from build123d import *

# Parameters (mm, degrees)
Y_KSEKLIK_EKSTR_ZYON1_DEPTH = 15
KES_EKSTR_ZYON1_DEPTH       = 10
IZIM4_W                     = 15
IZIM4_H                     = 10
KES_EKSTR_ZYON2_DEPTH       = 10


with BuildPart() as part:
    # Çizim2 → Yükseklik-Ekstrüzyon1 (new, symmetric)
    with BuildSketch(Plane.XY):
        Polygon((0, 0), (0, 30), (-10, 30), (-10, 10), (-40, 10), (-40, 0), align=None)
    extrude(amount=Y_KSEKLIK_EKSTR_ZYON1_DEPTH, both=True)

    # Çizim3 → Kes-Ekstrüzyon1 (cut)
    with BuildSketch(Plane(origin=(0, 0, 0), x_dir=(1, 0, 0), z_dir=(0, 1, 0))):
        Polygon((-40, 15), (-25, 15), (-40, 7.5), align=None)
        Polygon((-25, -15), (-40, -7.5), (-40, -15), align=None)
    extrude(amount=KES_EKSTR_ZYON1_DEPTH, mode=Mode.SUBTRACT)

    # Çizim4 → Kes-Ekstrüzyon2 (cut)
    with BuildSketch(Plane.ZY.offset(10)):
        with Locations((7.5, 25)):
            Rectangle(IZIM4_W, IZIM4_H)
    extrude(amount=-KES_EKSTR_ZYON2_DEPTH, mode=Mode.SUBTRACT)


solid = part.part
The model under review builds one solid part; all positions refer to its coordinate system, in mm. A direction names the side the tool comes from. Give positions to 0.01 mm unless a question says otherwise; leave off trailing zeros. Loops run counter-clockwise (first coordinate to the right, second up) from the corner with the lowest first, then second, coordinate; pieces in that order, holes last. Notation, with made-up numbers: (-7, 67) -> (38, 67) arc R10 ccw to (38, 75) -> close; hole circle Ø1 at (-40, 36.5). An arc over 180 degrees is marked (long way). Put each result on its own line as item: value. Start each with the question number.
1. We need section D-D on y = 12. State the section outline as (x, z) points.
2. We need section B-B on y = 4.5. State the section outline as (x, z) points.
3. We need section A-A on z = 11.75. State the section outline as (x, y) points, then the cut area to 3 significant figures.
4. We need section C-C on x = -25.5. State the section outline as (y, z) points.
5. Wall thickness on probe 1 along Y at (x, z) = (-38, -3); probe 2 along X at (y, z) = (27.5, -10.25); probe 3 along Y at (x, z) = (-1.5, 12.75): over which ranges is each line inside the solid? List them lowest first.
6. For faces 1 (the face through (-5, 25, 0)), 2 (the face through (-25, 10, 0)), 3 (the face through (-10, 8, 15)), list the 3-axis set-ups (+Z, -Z, +X, -X, +Y, -Y) from which the entire face can be reached by the end or side of a thin tool; tool diameter is ignored.
7. Clearance check with flat-ended pins moving along their axes: P1, Ø6, axis at y = 16, z = -4, coming from the +X side; P2, Ø3, axis at x = -5, y = 24, coming from the +Z side; P3, Ø10, axis at y = 19, z = 3.5, coming from the -X side; P4, Ø9, axis at x = -18, z = 4.5, coming from the +Y side. State where each tip first meets the part, or that it passes through.
Determined:
1. outline: (-10, -15) -> (0, -15) -> (0, 15) -> (-10, 15) -> close
2. outline: (-40, -7.5) -> (-25, -15) -> (0, -15) -> (0, 15) -> (-25, 15) -> (-40, 7.5) -> close
3. outline: (-31.5, 0) -> (0, 0) -> (0, 20) -> (-10, 20) -> (-10, 10) -> (-31.5, 10) -> close
3. area: 415 mm^2
4. outline: (0, -14.75) -> (10, -14.75) -> (10, 14.75) -> (0, 14.75) -> close
5. probe 1: 0 to 10
5. probe 2: -10 to 0
5. probe 3: 0 to 20
6. face 1: +Z, +X, -X, +Y
6. face 2: +Z, -Z, -X, +Y
6. face 3: +Z, +X, -X, +Y, -Y
7. P1: x = 0
7. P2: z = 0
7. P3: x = -10
7. P4: y = 10
